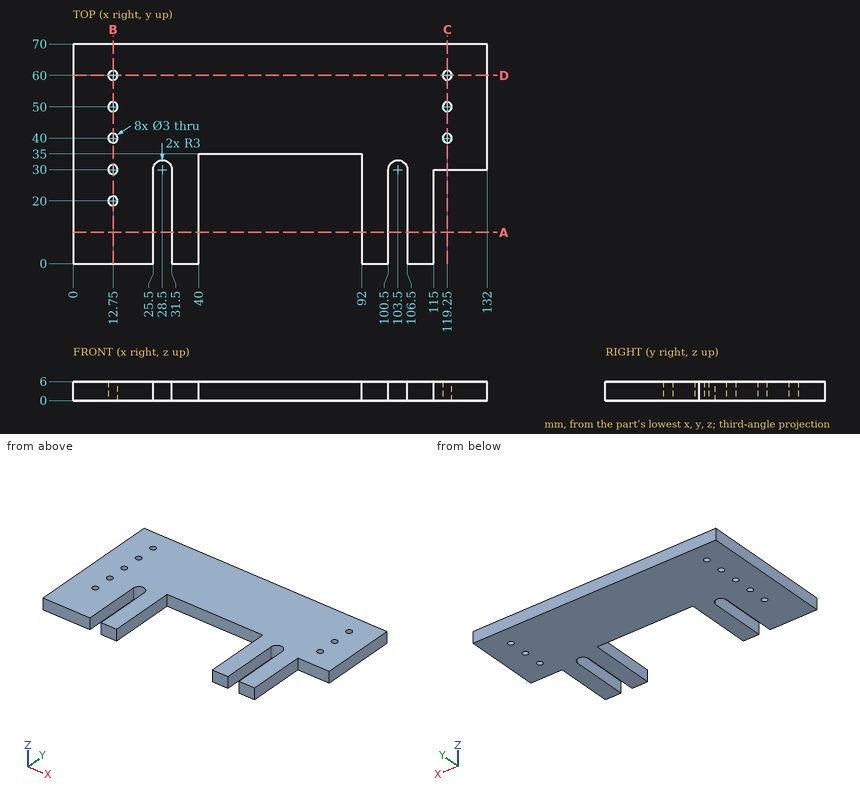
Print and shaded views of the part. All mm, measured from the part's lowest x, y and z. Give positions to 0.01 mm unless a question says otherwise; leave off trailing zeros. Order: outer loops, then holes, each group sorted by start corner. A loop starts at its lowest first (then second) coordinate and runs counter-clockwise, first axis right, second up. Notation, with made-up numbers: (38.5, -9.5) - (88.5, -9.5) arc R14 ccw to (88.5, 15.5) - close; hole circle Ø8 at (-4, 12). An arc over 180 degrees is marked (long way). One line per item, written item: value.
Item 1: Slice it at D-D (y = 60). List the corners of the cut face in (x, z), then the cut area to 3 significant figures.
Response values:
outline: (0, 0) - (11.25, 0) - (11.25, 6) - (0, 6) - close; (14.25, 0) - (117.75, 0) - (117.75, 6) - (14.25, 6) - close; (120.75, 0) - (132, 0) - (132, 6) - (120.75, 6) - close
area: 756 mm2
Item 2: Wall check: line 1 (Y direction, x = 12.75, z = 2.3); line 2 (X direction, y = 7.5, z = 3.35); line 3 (Y direction, x = 119.25, z = 3.9). Give the ranges that are in metal, low to high.
Response values:
line 1: 0 to 18.5, 21.5 to 28.5, 31.5 to 38.5, 41.5 to 48.5, 51.5 to 58.5, 61.5 to 70
line 2: 0 to 25.5, 31.5 to 40, 92 to 100.5, 106.5 to 115
line 3: 30 to 38.5, 41.5 to 48.5, 51.5 to 58.5, 61.5 to 70
Item 3: Slice it at A-A (y = 10). List the corners of the cut face in (x, z).
Response values:
outline: (0, 0) - (25.5, 0) - (25.5, 6) - (0, 6) - close; (31.5, 0) - (40, 0) - (40, 6) - (31.5, 6) - close; (92, 0) - (100.5, 0) - (100.5, 6) - (92, 6) - close; (106.5, 0) - (115, 0) - (115, 6) - (106.5, 6) - close
Item 4: Pin check, flat tips, straight feed: pin 1 Ø3 at (y, z) = (22, 2.5) entering from +X; pin 2 Ø1.8 at (x, z) = (65.5, 2) entering from -Y. Stop position of each tip, or through.
Response values:
pin 1: x = 115
pin 2: y = 35
Item 5: Slice it at B-B (x = 12.75). List the corners of the cut face in (y, z), then the cut area to 3 significant figures.
Response values:
outline: (0, 0) - (18.5, 0) - (18.5, 6) - (0, 6) - close; (21.5, 0) - (28.5, 0) - (28.5, 6) - (21.5, 6) - close; (31.5, 0) - (38.5, 0) - (38.5, 6) - (31.5, 6) - close; (41.5, 0) - (48.5, 0) - (48.5, 6) - (41.5, 6) - close; (51.5, 0) - (58.5, 0) - (58.5, 6) - (51.5, 6) - close; (61.5, 0) - (70, 0) - (70, 6) - (61.5, 6) - close
area: 330 mm2
Item 6: Slice it at C-C (x = 119.25). List the corners of the cut face in (y, z).
Response values:
outline: (30, 0) - (38.5, 0) - (38.5, 6) - (30, 6) - close; (41.5, 0) - (48.5, 0) - (48.5, 6) - (41.5, 6) - close; (51.5, 0) - (58.5, 0) - (58.5, 6) - (51.5, 6) - close; (61.5, 0) - (70, 0) - (70, 6) - (61.5, 6) - close
